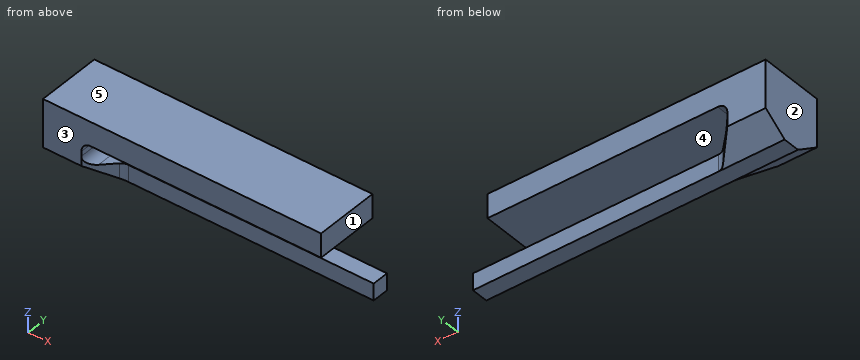
from build123d import *

# Parameters (mm, degrees)
SKETCH_1_W      = 60
SKETCH_1_H      = 3.5
EXTRUDE_1_DEPTH = 3.5
SKETCH_2_W      = 3
SKETCH_2_H      = 5
SKETCH_2_H_2    = 3.5
EXTRUDE_2_DEPTH = 10
EXTRUDE_3_DEPTH = 3
SKETCH_4_W      = 5
SKETCH_4_H      = 5.5
SKETCH_4_H_2    = 4
EXTRUDE_4_DEPTH = 50
CHAMFER_1_SIZE  = 5
FILLET_1_R      = 2
EXTRUDE_5_DEPTH = 5


# Some blends are built 0.0001 mm under size
with BuildPart() as part:
    # 草图1 → 凸台-拉伸1 (new body)
    with BuildSketch(Plane.XY):
        with Locations((15.433843148, 11.499032355)):
            Rectangle(SKETCH_1_W, SKETCH_1_H)
    extrude(amount=EXTRUDE_1_DEPTH)

    # 草图2 → 凸台-拉伸2 (add)
    with BuildSketch(Plane.XY.offset(3.5)):
        with Locations((-13.066156852, 15.749032355)):
            Rectangle(SKETCH_2_W, SKETCH_2_H)
        with Locations((-13.066156852, 11.499032355)):
            Rectangle(SKETCH_2_W, SKETCH_2_H_2)
        with Locations((-13.066156852, 7.249032355)):
            Rectangle(SKETCH_2_W, SKETCH_2_H)
    extrude(amount=EXTRUDE_2_DEPTH)

    # 草图3 → 凸台-拉伸3 (add)
    with BuildSketch(Plane.ZY.offset(14.566156852)):
        Polygon((0, 9.749032355), (3.5, 4.749032355), (3.5, 9.749032355), align=None)
        Polygon((3.5, 18.249032355), (0, 13.249032355), (3.5, 13.249032355), align=None)
    extrude(amount=-EXTRUDE_3_DEPTH)

    # 草图4 → 凸台-拉伸4 (add)
    with BuildSketch(Plane(origin=(-11.566156852, 0, 0), x_dir=(0, 0, -1), z_dir=(1, 0, 0))):
        with Locations((-11, 11.499032355)):
            Rectangle(SKETCH_4_W, SKETCH_4_H)
        with Locations((-11, 6.749032355)):
            Rectangle(SKETCH_4_W, SKETCH_4_H_2)
        with Locations((-11, 16.249032355)):
            Rectangle(SKETCH_4_W, SKETCH_4_H_2)
    extrude(amount=EXTRUDE_4_DEPTH)

    # 倒角1
    chamfer_1_edges = [part.edges().sort_by_distance(p)[0] for p in [
        (-11.566156852, 9.749032355, 1.75),
        (-11.566156852, 13.249032355, 1.75),
    ]]
    chamfer(chamfer_1_edges, length=CHAMFER_1_SIZE - 0.0001)  # a hair under: the kernel refuses the full size

    # 圆角1
    # the kernel refuses this fillet: 2 mm, written as the material it adds along each edge
    with BuildSketch(Plane(origin=(-11.566156852, 23.248932355, 3.5), x_dir=(1, 0, 0), z_dir=(0, -1, 0))) as fillet_1_piece_1_section:
        with BuildLine():
            CenterArc((FILLET_1_R, FILLET_1_R), FILLET_1_R, 180, 90)
            Line((0, FILLET_1_R), (0, 0))
            Line((0, 0), (FILLET_1_R, 0))
        make_face()
    fillet_1_piece_1 = extrude(amount=23.4998, mode=Mode.PRIVATE)
    fillet_1_piece_1 = split(fillet_1_piece_1, bisect_by=Plane(origin=(-7.979513836, 8.335775371, 3.970107375), z_dir=(-0.7071067811865476, 0.7071067811865476, 0)), keep=Keep.TOP, mode=Mode.PRIVATE)
    fillet_1_piece_1 = split(fillet_1_piece_1, bisect_by=Plane(origin=(-7.979513836, 14.662289339, 3.970107375), z_dir=(-0.7071067811865475, -0.7071067811865477, 0)), keep=Keep.TOP, mode=Mode.PRIVATE)
    fillet_1_piece_1 = split(fillet_1_piece_1, bisect_by=Plane(origin=(-11.14277082, 4.749032355, 3.970107375), z_dir=(0, 1, 0)), keep=Keep.TOP, mode=Mode.PRIVATE)
    fillet_1_piece_1 = split(fillet_1_piece_1, bisect_by=Plane(origin=(-11.14277082, 18.249032355, 3.970107375), z_dir=(0, -1, 0)), keep=Keep.TOP, mode=Mode.PRIVATE)
    fillet_1_piece_1 = split(fillet_1_piece_1, bisect_by=Plane(origin=(-11.14277082, 13.939686827, 0.48345813), z_dir=(0, -0.5734623443633282, 0.8192319205190406)), keep=Keep.TOP, mode=Mode.PRIVATE)
    add(fillet_1_piece_1)
    with BuildSketch(Plane(origin=(-11.566156852, 18.249032355, 8.5), x_dir=(0, 0, -1), z_dir=(0, -1, 0))) as fillet_1_piece_2:
        with BuildLine():
            CenterArc((FILLET_1_R, FILLET_1_R), FILLET_1_R, 180, 90)
            Line((0, FILLET_1_R), (0, 0))
            Line((0, 0), (FILLET_1_R, 0))
        make_face()
    extrude(amount=13.5)
    with BuildSketch(Plane(origin=(-6.566256852, 9.749032355, 3.5), x_dir=(-0.7071067811865475, -0.7071067811865475, 0), z_dir=(0, 0, -1))) as fillet_1_piece_3_section:
        with BuildLine():
            CenterArc((FILLET_1_R * 0.414213562373, -FILLET_1_R), FILLET_1_R, 90, 45)
            Line((-FILLET_1_R * 0.292893218813, -FILLET_1_R * 0.292893218813), (0, 0))
            Line((0, 0), (FILLET_1_R * 0.414213562373, 0))
        make_face()
    fillet_1_piece_3 = extrude(amount=3.5, mode=Mode.PRIVATE)
    fillet_1_piece_3 = split(fillet_1_piece_3, bisect_by=Plane(origin=(-6.5069765, 8.826534018, 0.645748836), z_dir=(0, 0.5734623443633283, 0.8192319205190405)), keep=Keep.TOP, mode=Mode.PRIVATE)
    add(fillet_1_piece_3)
    with BuildSketch(Plane(origin=(-6.566256852, 13.249032355, 0), x_dir=(1, 0, 0), z_dir=(0, 0, 1))) as fillet_1_piece_4_section:
        with BuildLine():
            CenterArc((FILLET_1_R * 0.414213562373, FILLET_1_R), FILLET_1_R, 225, 45)
            Line((-FILLET_1_R * 0.292893218813, FILLET_1_R * 0.292893218813), (0, 0))
            Line((0, 0), (FILLET_1_R * 0.414213562373, 0))
        make_face()
    fillet_1_piece_4 = extrude(amount=3.5, mode=Mode.PRIVATE)
    fillet_1_piece_4 = split(fillet_1_piece_4, bisect_by=Plane(origin=(-6.5069765, 14.171530692, 0.645748836), z_dir=(0, -0.5734623443633282, 0.8192319205190406)), keep=Keep.TOP, mode=Mode.PRIVATE)
    add(fillet_1_piece_4)

    # 草图5 → 凸台-拉伸5 (add)
    with BuildSketch(Plane.ZY.offset(14.566156852)):
        Polygon((3.5, 18.249032355), (0, 13.249032355), (0, 9.749032355), (3.5, 4.749032355), (13.5, 4.749032355), (13.5, 18.249032355), align=None)
    extrude(amount=EXTRUDE_5_DEPTH)


solid = part.part
Design review of the part built by this model. Coordinates are the model's own, in mm. Face numbers are marked on the shaded views. A direction names the side the tool comes from. Give positions to 0.01 mm unless a question says otherwise; leave off trailing zeros. Order: outer loops, then holes, each group sorted by start corner. A loop starts at its lowest first (then second) coordinate and runs counter-clockwise, first axis right, second up. Notation, with made-up numbers: (76.25, 78) - (124.25, 78) arc R29 ccw to (124.25, 103) - close; hole circle Ø6 at (62.5, 79). An arc over 180 degrees is marked (long way). Write item = value, one per line. Start each with the question number.
Q1. Mouldability with a two-part tool opening along Z and no side actions: class the marked faces 3, 4 and 5 as released by +Z, released by -Z, zero draft, split by the parting line, or undercut.
Q2. Clearance check with flat-ended pins moving along their axes: pin 1 Ø6 at (x, z) = (8.5, 3.5) entering from -Y; pin 2 Ø6 at (y, z) = (9, 9.5) entering from +X; pin 3 Ø2.5 at (y, z) = (14.5, 5.5) entering from +X. State where each tip first meets the part, or that it passes through.
Q3. We need section C-C on y = 7.5. State the section outline as (x, z) points, plus the area to 3 significant figures.
Q4. We need section D-D on x = 40. State the section outline as (y, z) points, plus the area to 4 significant figures.
Q5. We need section B-B on z = 11.25. State the section outline as (x, y) points, plus the area to 3 significant figures.
Q6. Tool access review of the marked faces 1 and 2: name each direction out of +Z, -Z, +X, -X, +Y, -Y from which nothing blocks a thin tool from reaching the whole face with its end or side.
Q7. We need section A-A on x = 31.5. State the section outline as (y, z) points, plus the area to 4 significant figures.
Q8. To check wall thickness, follow L1, parallel to Z at x = 10.5, y = 10.5; L2, parallel to Y at x = 34, z = 2.25; L3, parallel to X at y = 7, z = 6.25. State the ranges of each line that lie inside material, in increasing order. Write a range as from..to.
Working result:
q1.face_3 = zero draft
q1.face_4 = undercut
q1.face_5 = released by +Z
q2.pin_1 = 9.75
q2.pin_2 = 38.43
q2.pin_3 = -11.13
q3.outline = (-19.57, 1.57) - (-8.82, 1.57) - (-8.82, 3.5) - (-9.57, 3.5) arc R2 cw to (-11.57, 5.5) - (-11.57, 6.5) arc R2 cw to (-9.57, 8.5) - (38.43, 8.5) - (38.43, 13.5) - (-19.57, 13.5) - close
q3.area = 352 mm²
q4.outline = (9.75, 0) - (13.25, 0) - (13.25, 3.5) - (9.75, 3.5) - close
q4.area = 12.25 mm²
q5.outline = (-19.57, 4.75) - (38.43, 4.75) - (38.43, 18.25) - (-19.57, 18.25) - close
q5.area = 783 mm²
q6.face_1 = +Z, +X, +Y, -Y
q6.face_2 = +Z, -Z, -X, +Y, -Y
q7.outline = (4.75, 8.5) - (18.25, 8.5) - (18.25, 13.5) - (4.75, 13.5) - close; (9.75, 0) - (13.25, 0) - (13.25, 3.5) - (9.75, 3.5) - close
q7.area = 79.75 mm²
q8.L1 = 0..3.5, 8.5..13.5
q8.L2 = 9.75..13.25
q8.L3 = -19.57..-11.57
